For this review, take the finished solid that the model builds, in its own axes (mm). Face numbers are marked on the shaded views. Round coordinates to 2 decimals unless told otherwise and drop trailing zeros. Loops run counter-clockwise (first coordinate to the right, second up) from the corner with the lowest first, then second, coordinate; pieces in that order, holes last.
1. Draft analysis for pull direction Y (two halves, no side actions). For the marked faces 1 and 2, state which applies: released by +Y, released by -Y, zero draft, split by the parting line, or undercut.
2. Consider section C-C on z = 56.1. State the section outline as (x, y) points.
3. Consider section D-D on y = 45.5. State the section outline as (x, z) points, then the cut area to 4 significant figures.
4. Consider section B-B on y = 82.5. State the section outline as (x, z) points, then the cut area to 4 significant figures.
5. To check wall thickness, follow line 1 along Y through (x, z) = (5, 103); line 2 along Y through (x, z) = (1.5, 56.1); line 3 along Z through (x, y) = (7.5, 24.5). State the ranges of each line that lie inside material, in increasing order.
6. Clearance check with flat-ended pins moving along their axes: pin 1 Ø8 at (y, z) = (68, 92.5) entering from -X; pin 2 Ø1.5 at (x, y) = (2.5, 32.5) entering from -Z; pin 3 Ø4 at (y, z) = (13.5, 98.1) entering from +X. State where each tip first meets the part, or that it passes through.
7. Consider section A-A on y = 59. State the section outline as (x, z) points, then the cut area to 3 significant figures.
from build123d import *
from build123d.topology import SkipClean

# Parameters (mm, degrees)
SKETCH1_W                    = 81
SKETCH1_H                    = 83
BODY_DEPTH                   = 8.5
RAILFILLET_R                 = 1
FOOTCHAMFER_SIZE             = 1
SKETCH5_W                    = 81
SKETCH5_H                    = 83
BOSS_EXTRUDE3_DEPTH          = 8.5
SKETCH6_W                    = 93
SKETCH6_H                    = 97
CUT_EXTRUDE3_DEPTH           = 6
F_8_36_TAPPED_HOLE1_D        = 3.4544
F_8_36_TAPPED_HOLE1_DEPTH    = 13.55
F_8_36_TAPPED_HOLE1_TIP      = 1.037806461
SKETCH57_W                   = 1
SKETCH57_H                   = 4
BOSS_EXTRUDE24_DEPTH         = 6
FILLET5_R                    = 4
M3X0_5_TAPPED_HOLE1_D        = 2.5
FILLET7_R                    = 4
M3X0_5_TAPPED_HOLE2_D        = 2.5
M3X0_5_TAPPED_HOLE2_DEPTH    = 7.5
M3X0_5_TAPPED_HOLE2_TIP      = 0.751075774
FILLET8_R                    = 4
SKETCH70_R                   = 4
CUT_EXTRUDE14_DEPTH          = 1.5
SKETCH75_W                   = 7.5
SKETCH75_H                   = 4
BOSS_EXTRUDE25_DEPTH         = 1.4
M1_6X0_35_TAPPED_HOLE1_D     = 1.25
M1_6X0_35_TAPPED_HOLE1_DEPTH = 4.25
M1_6X0_35_TAPPED_HOLE1_TIP   = 0.375537887
FILLET9_R                    = 4
F_1_5MM_DOWEL_HOLE1_REACH    = 153.507
F_1_5MM_DOWEL_HOLE1_BORE_R   = 0.75
CUT_EXTRUDE15_DEPTH          = 152.387747196
SKETCH84_R                   = 1.75
CUT_EXTRUDE17_DEPTH          = 152.507425566


# Some blends are built 0.0001 mm under size
with BuildPart() as part:
    # Sketch1 → Body (new body)
    with BuildSketch(Plane(origin=(0, 0, 0), x_dir=(0, 0, -1), z_dir=(1, 0, 0))):
        Polygon((-113.5, 0), (0, 0), (0, 8.5), (-7.5, 8.5), (-7.5, 91.5), (0, 91.5), (0, 100), (-113.5, 100), (-113.5, 91.5), (-104.5, 91.5), (-104.5, 8.5), (-113.5, 8.5), align=None)
        with Locations((-56, 50)):
            Rectangle(SKETCH1_W, SKETCH1_H, mode=Mode.SUBTRACT)
    extrude(amount=BODY_DEPTH)

    # RailFillet
    railfillet_edges = [part.edges().sort_by_distance(p)[0] for p in [
        (0, 0, 56.75),
        (0, 100, 56.75),
    ]]
    fillet(railfillet_edges, radius=RAILFILLET_R)

    # FootChamfer
    footchamfer_edges = [part.edges().sort_by_distance(p)[0] for p in [
        (8.5, 95.75, 0),
        (0, 95.25, 113.5),
        (8.5, 95.75, 113.5),
        (0, 95.25, 0),
        (4.25, 8.5, 0),
        (4.75, 0, 0),
        (4.75, 0, 113.5),
        (4.25, 8.5, 113.5),
        (4.25, 91.5, 113.5),
        (4.75, 100, 113.5),
        (4.75, 100, 0),
        (4.25, 91.5, 0),
        (8.5, 4.25, 113.5),
        (8.5, 4.25, 0),
        (0, 4.75, 0),
        (0, 4.75, 113.5),
        (0.292893219, 0.292893219, 113.5),
        (0.292893219, 0.292893219, 0),
        (0.292893219, 99.707106781, 113.5),
        (0.292893219, 99.707106781, 0),
    ]]
    chamfer(footchamfer_edges, length=FOOTCHAMFER_SIZE - 0.0001)  # a hair under: the kernel refuses the full size

    # Sketch5 → Boss-Extrude3 (add)
    with BuildSketch(Plane(origin=(8.5, 0, 0), x_dir=(0, 0, -1), z_dir=(1, 0, 0))):
        with Locations((-56, 50)):
            Rectangle(SKETCH5_W, SKETCH5_H)
    extrude(amount=-BOSS_EXTRUDE3_DEPTH)

    # Sketch6 → Cut-Extrude3 (cut)
    with BuildSketch(Plane(origin=(8.5, 0, 0), x_dir=(0, 0, -1), z_dir=(1, 0, 0))):
        with Locations((-56, 50)):
            Rectangle(SKETCH6_W, SKETCH6_H)
    extrude(amount=-CUT_EXTRUDE3_DEPTH, mode=Mode.SUBTRACT)

    # #8-36 Tapped Hole1
    with Locations(Plane(origin=(0, 0, 0), x_dir=(-1, 0, 0), z_dir=(0, 0, -1))):
        with Locations((-4.25, 95.75)):
            Hole(F_8_36_TAPPED_HOLE1_D / 2, depth=F_8_36_TAPPED_HOLE1_DEPTH)
            with Locations((0, 0, -(F_8_36_TAPPED_HOLE1_DEPTH + F_8_36_TAPPED_HOLE1_TIP / 2))):  # 118° drill point
                Cone(0, F_8_36_TAPPED_HOLE1_D / 2, F_8_36_TAPPED_HOLE1_TIP, mode=Mode.SUBTRACT)

    # Sketch57 → Boss-Extrude24 (add)
    with BuildSketch(Plane(origin=(2.5, 0, 0), x_dir=(0, 0, -1), z_dir=(1, 0, 0))):
        with Locations((-102, 82.5)):
            Rectangle(SKETCH57_W, SKETCH57_H)
        with Locations((-102, 17.5)):
            Rectangle(SKETCH57_W, SKETCH57_H)
        with Locations((-10, 17.5)):
            Rectangle(SKETCH57_W, SKETCH57_H)
        with Locations((-10, 82.5)):
            Rectangle(SKETCH57_W, SKETCH57_H)
    extrude(amount=BOSS_EXTRUDE24_DEPTH)

    # Fillet5
    # the kernel refuses this fillet: 4 mm, written as the material it adds along each edge
    with BuildSketch(Plane(origin=(2.5, 84.5, 102.5), x_dir=(0, 1, 0), z_dir=(1, 0, 0)), Plane(origin=(2.5, 19.5, 102.5), x_dir=(0, 1, 0), z_dir=(1, 0, 0)), Plane(origin=(2.5, 15.5, 9.5), x_dir=(0, -1, 0), z_dir=(1, 0, 0)), Plane(origin=(2.5, 80.5, 9.5), x_dir=(0, -1, 0), z_dir=(1, 0, 0))) as fillet5_piece_1:
        with BuildLine():
            CenterArc((2.645751311, -4), FILLET5_R, 90, 41.409622109)
            Line((0, -1), (-0.052915026, -0.94))
            ThreePointArc((-0.052915026, -0.94), (-0.08, -0.5), (-0.08, 0))
            Line((-0.08, 0), (0, 0.08))
            Line((0, 0.08), (2.645751311, 0.08))
            Line((2.645751311, 0.08), (2.645751311, 0))
        make_face()
    extrude(amount=6)
    with BuildSketch(Plane(origin=(2.5, 80.5, 102.5), x_dir=(0, -1, 0), z_dir=(1, 0, 0)), Plane(origin=(2.5, 15.5, 102.5), x_dir=(0, -1, 0), z_dir=(1, 0, 0)), Plane(origin=(2.5, 19.5, 9.5), x_dir=(0, 1, 0), z_dir=(1, 0, 0)), Plane(origin=(2.5, 84.5, 9.5), x_dir=(0, 1, 0), z_dir=(1, 0, 0))) as fillet5_piece_2:
        with BuildLine():
            CenterArc((2.645751311, 4), FILLET5_R, 228.590377891, 41.409622109)
            Line((0, 1), (-0.052915026, 0.94))
            ThreePointArc((-0.052915026, 0.94), (-0.08, 0.5), (-0.08, 0))
            Line((-0.08, 0), (0, -0.08))
            Line((0, -0.08), (2.645751311, -0.08))
            Line((2.645751311, -0.08), (2.645751311, 0))
        make_face()
    extrude(amount=6)

    # M3x0.5 Tapped Hole1 (through all)
    with Locations(Plane(origin=(0, 0, 7.5), x_dir=(-1, 0, 0), z_dir=(0, 0, -1))):
        with Locations((-5, 82.5), (-5, 17.5)):
            Hole(M3X0_5_TAPPED_HOLE1_D / 2)

    # Fillet7
    # the kernel refuses this fillet: 4 mm, written as the material it adds along each edge
    with BuildSketch(Plane(origin=(8.5, 1.5, 102.5), x_dir=(0, 1, 0), z_dir=(-1, 0, 0)), Plane(origin=(8.5, 98.5, 102.5), x_dir=(0, 0, -1), z_dir=(-1, 0, 0)), Plane(origin=(8.5, 1.5, 9.5), x_dir=(0, 0, 1), z_dir=(-1, 0, 0))) as fillet7_piece_1:
        with BuildLine():
            CenterArc((FILLET7_R, FILLET7_R), FILLET7_R, 180, 90)
            Line((0, FILLET7_R), (0, 0))
            Line((0, 0), (FILLET7_R, 0))
        make_face()
    extrude(amount=6)
    with BuildSketch(Plane(origin=(8.5, 98.5, 9.5), x_dir=(0, -1, 0), z_dir=(-1, 0, 0))) as fillet7_piece_2_section:
        with BuildLine():
            CenterArc((FILLET7_R, FILLET7_R), FILLET7_R, 180, 90)
            Line((0, FILLET7_R), (0, 0))
            Line((0, 0), (FILLET7_R, 0))
        make_face()
    fillet7_piece_2 = extrude(amount=6, mode=Mode.PRIVATE)
    fillet7_piece_2 = fillet7_piece_2 - Plane(origin=(4.25, 95.75, 10.518489618), x_dir=(1, 0, 0), z_dir=(0, 0, 1)) * Cylinder(1.7272, 28, mode=Mode.PRIVATE)
    add(fillet7_piece_2)

    # M3x0.5 Tapped Hole2
    with Locations(Plane.ZY):
        with Locations((14.1, 13.5), (14.1, 86.5), (98.1, 86.5), (98.1, 13.5)):
            Hole(M3X0_5_TAPPED_HOLE2_D / 2, depth=M3X0_5_TAPPED_HOLE2_DEPTH)
            with Locations((0, 0, -(M3X0_5_TAPPED_HOLE2_DEPTH + M3X0_5_TAPPED_HOLE2_TIP / 2))):  # 118° drill point
                Cone(0, M3X0_5_TAPPED_HOLE2_D / 2, M3X0_5_TAPPED_HOLE2_TIP, mode=Mode.SUBTRACT)

    # Fillet8
    fillet8_edges = [part.edges().sort_by_distance(p)[0] for p in [
        (4.25, 8.5, 7.5),
        (4.25, 8.5, 104.5),
        (4.25, 91.5, 104.5),
        (4.25, 91.5, 7.5),
    ]]
    fillet(fillet8_edges, radius=FILLET8_R)

    # Sketch70 → Cut-Extrude14 (cut)
    with BuildSketch(Plane(origin=(2.5, 0, 0), x_dir=(0, 0, -1), z_dir=(1, 0, 0))):
        with BuildLine():
            ThreePointArc((-13.5, 1.5), (-9.5, 5.5), (-13.5, 9.5))
            Line((-13.5, 9.5), (-28.5, 9.5))
            ThreePointArc((-28.5, 9.5), (-32.5, 5.5), (-28.5, 1.5))
            Line((-28.5, 1.5), (-13.5, 1.5))
        make_face()
        with Locations((-13.5, 94.5)):
            Circle(SKETCH70_R)
    extrude(amount=-CUT_EXTRUDE14_DEPTH, mode=Mode.SUBTRACT)

    # Sketch75 → Boss-Extrude25 (add)
    with BuildSketch(Plane(origin=(0, 1.5, 0), x_dir=(1, 0, 0), z_dir=(0, 1, 0))):
        with Locations((4.75, -22.5)):
            Rectangle(SKETCH75_W, SKETCH75_H)
    extrude(amount=BOSS_EXTRUDE25_DEPTH)

    # M1.6x0.35 Tapped Hole1
    with Locations(Plane(origin=(0, 2.9, 0), x_dir=(1, 0, 0), z_dir=(0, 1, 0))):
        with Locations((3.3, -22.5), (7.3, -22.5)):
            Hole(M1_6X0_35_TAPPED_HOLE1_D / 2, depth=M1_6X0_35_TAPPED_HOLE1_DEPTH)
            with Locations((0, 0, -(M1_6X0_35_TAPPED_HOLE1_DEPTH + M1_6X0_35_TAPPED_HOLE1_TIP / 2))):  # 118° drill point
                Cone(0, M1_6X0_35_TAPPED_HOLE1_D / 2, M1_6X0_35_TAPPED_HOLE1_TIP, mode=Mode.SUBTRACT)

    # Fillet9
    # the kernel refuses this fillet: 4 mm, written as the material it adds along each edge
    with BuildSketch(Plane(origin=(8.5, 1.5, 24.5), x_dir=(0, 1, 0), z_dir=(-1, 0, 0))) as fillet9_piece_1:
        with BuildLine():
            CenterArc((4, -3.039736831), FILLET9_R, 130.541601874, 49.458398126)
            Line((0, -3.039736831), (-0.08, -3.039736831))
            Line((-0.08, -3.039736831), (-0.08, 0))
            Line((-0.08, 0), (0, 0.08))
            ThreePointArc((0, 0.08), (0.7, 0.08), (1.348, 0.060794737))
            Line((1.348, 0.060794737), (1.4, 0))
        make_face()
    extrude(amount=6)
    with BuildSketch(Plane(origin=(2.5, 1.5, 20.5), x_dir=(0, 0, -1), z_dir=(1, 0, 0))) as fillet9_piece_2:
        with BuildLine():
            CenterArc((3.039736831, 4), FILLET9_R, 220.541601874, 49.458398126)
            Line((0, 1.4), (-0.060794737, 1.348))
            ThreePointArc((-0.060794737, 1.348), (-0.08, 0.7), (-0.08, 0))
            Line((-0.08, 0), (0, -0.08))
            Line((0, -0.08), (3.039736831, -0.08))
            Line((3.039736831, -0.08), (3.039736831, 0))
        make_face()
    extrude(amount=6)
    with BuildSketch(Plane(origin=(1, 1.5, 20.5), x_dir=(0, 1, 0), z_dir=(1, 0, 0)), Plane(origin=(2.5, 1.5, 24.5), x_dir=(0, 1, 0), z_dir=(-1, 0, 0))) as fillet9_piece_3:
        with BuildLine():
            CenterArc((4, -3.039736831), FILLET9_R, 130.541601874, 49.458398126)
            Line((0, -3.039736831), (-0.08, -3.039736831))
            Line((-0.08, -3.039736831), (-0.08, 0))
            Line((-0.08, 0), (0, 0.08))
            ThreePointArc((0, 0.08), (0.7, 0.08), (1.348, 0.060794737))
            Line((1.348, 0.060794737), (1.4, 0))
        make_face()
    extrude(amount=1.5)

    # Ø1.5mm Dowel Hole1 bore → Ø1.5mm Dowel Hole1 (cut, up to next)
    with BuildSketch(Plane(origin=(0, 0, 0), x_dir=(-1, 0, 0), z_dir=(0, 0, -1)), mode=Mode.PRIVATE) as f_1_5mm_dowel_hole1_sk1:
        with Locations((-4.25, 4.25)):
            Circle(F_1_5MM_DOWEL_HOLE1_BORE_R)
    f_1_5mm_dowel_hole1_tool1 = extrude(f_1_5mm_dowel_hole1_sk1.sketch, amount=-F_1_5MM_DOWEL_HOLE1_REACH, mode=Mode.PRIVATE) & part.part
    add(f_1_5mm_dowel_hole1_tool1.solids().sort_by_distance((4.25, 4.25, 0))[0], mode=Mode.SUBTRACT)

    # Sketch81 → Cut-Extrude15 (cut, through all)
    with SkipClean():  # the faces are left unmerged after this step: merging them gives an invalid solid
        with BuildSketch(Plane(origin=(2.5, 0, 0), x_dir=(0, 0, -1), z_dir=(1, 0, 0))):
            with BuildLine():
                ThreePointArc((-102.5, 51.5), (-101.914213562, 50.085786438), (-100.5, 49.5))
                ThreePointArc((-100.5, 49.5), (-99.085786438, 50.085786438), (-98.5, 51.5))
                Line((-98.5, 51.5), (-98.5, 76.5))
                ThreePointArc((-98.5, 76.5), (-99.085786438, 77.914213562), (-100.5, 78.5))
                ThreePointArc((-100.5, 78.5), (-101.914213562, 77.914213562), (-102.5, 76.5))
                Line((-102.5, 76.5), (-102.5, 51.5))
            make_face()
            with BuildLine():
                Line((-85.1, 51.5), (-85.1, 76.5))
                ThreePointArc((-85.1, 76.5), (-87.1, 78.5), (-89.1, 76.5))
                Line((-89.1, 76.5), (-89.1, 51.5))
                ThreePointArc((-89.1, 51.5), (-87.1, 49.5), (-85.1, 51.5))
            make_face()
            with BuildLine():
                ThreePointArc((-87.1, 49.5), (-88.514213562, 50.085786438), (-89.1, 51.5))
                Line((-89.1, 51.5), (-89.1, 76.5))
                ThreePointArc((-89.1, 76.5), (-88.514213562, 77.914213562), (-87.1, 78.5))
                Line((-87.1, 78.5), (-100.5, 78.5))
                ThreePointArc((-100.5, 78.5), (-99.085786438, 77.914213562), (-98.5, 76.5))
                Line((-98.5, 76.5), (-98.5, 51.5))
                ThreePointArc((-98.5, 51.5), (-99.085786438, 50.085786438), (-100.5, 49.5))
                Line((-100.5, 49.5), (-87.1, 49.5))
            make_face()
        extrude(amount=-CUT_EXTRUDE15_DEPTH, mode=Mode.SUBTRACT)

    # Sketch84 → Cut-Extrude17 (cut, through all)
    with SkipClean():  # the faces are left unmerged after this step: merging them gives an invalid solid
        with BuildSketch(Plane.ZY):
            with Locations((56.1, 36)):
                Circle(SKETCH84_R)
            with Locations((56.1, 64)):
                Circle(SKETCH84_R)
        extrude(amount=-CUT_EXTRUDE17_DEPTH, mode=Mode.SUBTRACT)


solid = part.part
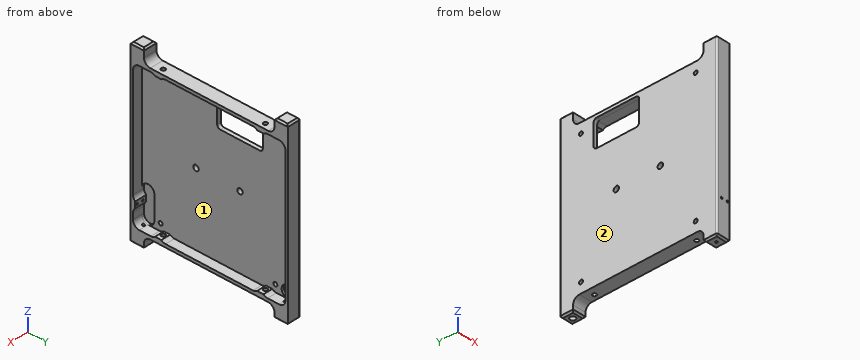
Resolved:
1. face 1: undercut
1. face 2: zero draft
2. outline: (0, 1) arc R1 ccw to (1, 0) - (8.5, 0) - (8.5, 1.5) - (2.5, 1.5) - (2.5, 34.25) - (0, 34.25) - close; (0, 37.75) - (2.5, 37.75) - (2.5, 62.25) - (0, 62.25) - close; (0, 65.75) - (2.5, 65.75) - (2.5, 98.5) - (8.5, 98.5) - (8.5, 100) - (1, 100) arc R1 ccw to (0, 99) - close
3. outline: (0, 7.5) - (8.5, 7.5) - (8.5, 9.5) - (2.5, 9.5) - (2.5, 102.5) - (8.5, 102.5) - (8.5, 104.5) - (0, 104.5) - close
3. area: 266.5 mm2
4. outline: (0, 7.5) - (3.75, 7.5) - (3.75, 10.5) - (2.5, 10.5) - (2.5, 101.5) - (3.75, 101.5) - (3.75, 104.5) - (0, 104.5) - close; (6.25, 7.5) - (8.5, 7.5) - (8.5, 10.5) - (6.25, 10.5) - close; (6.25, 101.5) - (8.5, 101.5) - (8.5, 104.5) - (6.25, 104.5) - close
4. area: 263.5 mm2
5. line 1: y = 0 to 16.25, 18.75 to 81.25, 83.75 to 100
5. line 2: y = 0 to 34.25, 37.75 to 62.25, 65.75 to 100
5. line 3: z = 7.5 to 9.5, 102.5 to 104.5
6. pin 1: passes through
6. pin 2: stops at z = 7.5
6. pin 3: stops at x = 2.5
7. outline: (0, 7.5) - (8.5, 7.5) - (8.5, 9.5) - (2.5, 9.5) - (2.5, 85.1) - (0, 85.1) - close; (0, 102.5) - (8.5, 102.5) - (8.5, 104.5) - (0, 104.5) - close
7. area: 223 mm2
